```python
from build123d import *

# Parameters (mm, degrees)
SKETCH1_R           = 14.4
SKETCH1_R_2         = 12.695
BOSS_EXTRUDE1_DEPTH = 39.37
BOSS_EXTRUDE2_START = -39.37
BOSS_EXTRUDE2_DEPTH = 39.37
CIRPATTERN1_COUNT   = 8
SKETCH3_OUTSIDE_W   = 48.978
SKETCH3_OUTSIDE_H   = 48.978
SKETCH3_OUTSIDE_R   = 14.255
CUT_EXTRUDE1_DEPTH  = 2.2
CHAMFER2_SIZE       = 0.25


with BuildPart() as part:
    # Sketch1 → Boss-Extrude1 (new body)
    with BuildSketch(Plane.XY):
        Circle(SKETCH1_R)
        Circle(SKETCH1_R_2, mode=Mode.SUBTRACT)
    extrude(amount=BOSS_EXTRUDE1_DEPTH)

    # Sketch2 → Boss-Extrude2 (add)
    with BuildSketch(Plane.XY.offset(39.37).offset(BOSS_EXTRUDE2_START)):
        with BuildLine():
            Line((-3.25, 16.915617784), (-3.25, 14.028453229))
            ThreePointArc((-3.25, 14.028453229), (0, 14.4), (3.25, 14.028453229))
            Line((3.25, 14.028453229), (3.25, 16.915617784))
            ThreePointArc((3.25, 16.915617784), (0, 17.225), (-3.25, 16.915617784))
        make_face()
    boss_extrude2 = extrude(amount=BOSS_EXTRUDE2_DEPTH)

    # CirPattern1: Boss-Extrude2 ×8 about axis
    cirpattern1_axis = Axis((0, 0, 0), (0, 0, 1))
    for i in range(1, CIRPATTERN1_COUNT):
        add(boss_extrude2.rotate(cirpattern1_axis, i * 360 / CIRPATTERN1_COUNT))

    # Sketch3 outside → Cut-Extrude1 (cut)
    with BuildSketch(Plane.XY.offset(39.37)):
        Rectangle(SKETCH3_OUTSIDE_W, SKETCH3_OUTSIDE_H)
        Circle(SKETCH3_OUTSIDE_R, mode=Mode.SUBTRACT)
    extrude(amount=-CUT_EXTRUDE1_DEPTH, mode=Mode.SUBTRACT)

    # Sketch5 → Cut-Revolve1 (revolve, cut)
    with BuildSketch(Plane(origin=(0, 0, 0), x_dir=(0, 0, -1), z_dir=(1, 0, 0))):
        Polygon((-35.67, 17.225), (-37.17, 15.725), (-37.17, 17.225), align=None)
        Polygon((0, 17.225), (-1.5, 17.225), (0, 15.725), align=None)
    revolve(axis=Axis((0, 0, 0), (0, 0, -1)), mode=Mode.SUBTRACT)

    # Sketch8 → Cut-Revolve2 (revolve, cut)
    with BuildSketch(Plane(origin=(0, 0, 0), x_dir=(1, 0, 0), z_dir=(0, 1, 0))):
        Polygon((-8.195, -5), (-8.195, 0), (-12.695, 0), (-12.695, -0.5), align=None)
        Polygon((-12.695, -0.5), (-12.695, 0), (-13.195, 0), align=None)
    revolve(axis=Axis((0, 0, 0), (0, 0, -1)), mode=Mode.SUBTRACT)

    # Chamfer2
    chamfer2_edges = [part.edges().sort_by_distance(p)[0] for p in [
        (-14.255, 0, 39.37),
        (-12.695, 0, 39.37),
    ]]
    chamfer(chamfer2_edges, length=CHAMFER2_SIZE)


solid = part.part
```
The listing builds one solid part. Answer for the finished solid, in the listing's coordinates (mm). A direction names the side the tool comes from. Coordinates: 2 decimals unless noted, no trailing zeros. Order: outer loops, then holes, each group sorted by start corner. A loop starts at its lowest first (then second) coordinate and runs counter-clockwise, first axis right, second up. Notation, with made-up numbers: M -26.75,52 L 20.25,52 A25 ccw 20.25,77 Z; hole C 16.5,38.25 d6. An arc over 180 degrees is marked long. Answer as a JSON object with one key per item and string values. Group by question number.
1. A tool of negligible diameter and unlimited length cuts with its end or side. For faces 5 (the cylindrical face through (5.48, -13.317, 18.325)), 6 (the conical face through (-16.464, -0.048, 36.43)), 7 (the cylindrical face through (13.317, 5.48, 18.325)), from which of +Z, -Z, +X, -X, +Y, -Y can it reach the whole face along a straight path? Write none if from no direction.
2. Straight lines are drawn through the part: line 1 (X direction, y = 0, z = 13) (3 decimals); line 2 (X direction, y = 13, z = 35.5); line 3 (X direction, y = 14.5, z = 20). For each, find the intervals that lie inside material, in ascending order.
3. Determine the mould class of faces 1 (the cylindrical face through (5.54, 13.29, 18.32)), 2 (the conical face through (11.676, -11.608, 0.739)), 3 (the cylindrical face through (-0.046, -17.225, 18.346)), 4 (the cylindrical face through (-10.074, -7.725, 19.54)) for opening direction X: released by +X, released by -X, zero draft, split by the parting line, or undercut.
4. Section A-A on x = 0 is taken. Write down the section's boundary in (y, z) (3 decimals), then the cut area to 3 significant figures.
5. Flat-ended cylindrical pins translate along their axes: P1, Ø1.4, axis at x = 16, z = 23.5, coming from the +Y side; P2, Ø1.4, axis at x = -16, z = 13.5, coming from the -Y side; P3, Ø1, axis at x = 11, y = 10, coming from the +Z side; P4, Ø15.5, axis at x = 3, y = -3, coming from the +Z side. Find the tip coordinate at first contact, or state that the pin passes through.
Values follow:
{
 "1": {"face 5": "+Z, -Z, -Y", "face 6": "+Z, -X", "face 7": "+Z, -Z, +X"},
 "2": {"line 1": "-17.225 to -12.695, 12.695 to 17.225", "line 2": "-11.3 to -8.4, -6.19 to 6.19, 8.4 to 11.3", "line 3": "-3.25 to 3.25"},
 "3": {"face 1": "undercut", "face 2": "released by +X", "face 3": "split by the parting line", "face 4": "undercut"},
 "4": {"outline": "M -17.225,1.5 L -15.725,0 L -13.195,0 L -12.695,0.5 L -12.695,39.12 L -12.945,39.37 L -14.005,39.37 L -14.255,39.12 L -14.255,37.17 L -15.725,37.17 L -17.225,35.67 Z; M 12.695,0.5 L 13.195,0 L 15.725,0 L 17.225,1.5 L 17.225,35.67 L 15.725,37.17 L 14.255,37.17 L 14.255,39.12 L 14.005,39.37 L 12.945,39.37 L 12.695,39.12 Z", "area": "339 mm2"},
 "5": {"P1": "y = 3.25", "P2": "y = -3.25", "P3": "z = 37.17", "P4": "through"}
}
